Could you check a few things on this model? Use its own coordinates, in mm. Face numbers are marked on the shaded views. A direction names the side the tool comes from. Round coordinates to 2 decimals unless told otherwise and drop trailing zeros. Loops run counter-clockwise (first coordinate to the right, second up) from the corner with the lowest first, then second, coordinate; pieces in that order, holes last. Notation, with made-up numbers: M 30,-32.5 L 66,-32.5 A24 cw 66,4.5 Z; hole C -9,31 d10. An arc over 180 degrees is marked long. One line per item, written item: value. Start each with the question number.
Q1. Imagine slicing it at C-C (x = 80). Please give me the cut outline in (y, z) (3 decimals).
Q2. Which directions (+Z, -Z, +X, -X, +Y, -Y) give clear straight access to the entire face, cutting with the end or side of a thin tool? Please do the marked faces 1, 2 and 3.
Q3. Imagine slicing it at D-D (x = 158). Please give me the cut outline in (y, z).
Q4. Imagine slicing it at A-A (y = 0). Please give me the cut outline in (x, z) (3 decimals), then the cut area to 3 significant figures.
Q5. I'm going to push flat-ended pins straight in: pin 1 Ø12 at (y, z) = (5, 10.5) entering from -X; pin 2 Ø10 at (x, z) = (220, -5.5) entering from +Y; pin 3 Ø1 at (x, y) = (141.5, -11) entering from -Z; pin 4 Ø1.5 at (y, z) = (6, -13) entering from +X. Where does each tip first touch, or does it pass through?
Q6. Please list where these lines run through material, in increasing order: line 1 along Y through (x, z) = (157, -10); line 2 along X through (y, z) = (11.5, -3).
from build123d import *


with BuildPart() as part:
    # Sketch1 → Revolve1 (revolve)
    with BuildSketch(Plane.XY):
        with BuildLine():
            Line((0, 0), (0, 7.5))
            Line((0, 7.5), (18.5, 7.5))
            ThreePointArc((18.5, 7.5), (19.560660172, 7.939339828), (20, 9))
            Line((20, 9), (20, 16.675))
            Line((20, 16.675), (142, 16.675))
            Line((142, 16.675), (142, 14))
            ThreePointArc((142, 14), (142.439339828, 12.939339828), (143.5, 12.5))
            Line((143.5, 12.5), (310, 12.5))
            Line((310, 12.5), (310, 9))
            ThreePointArc((310, 9), (310.439339828, 7.939339828), (311.5, 7.5))
            Line((311.5, 7.5), (330, 7.5))
            Line((330, 7.5), (330, 0))
            Line((330, 0), (0, 0))
        make_face()
    revolve(axis=Axis((330, 0, 0), (-1, 0, 0)))


solid = part.part
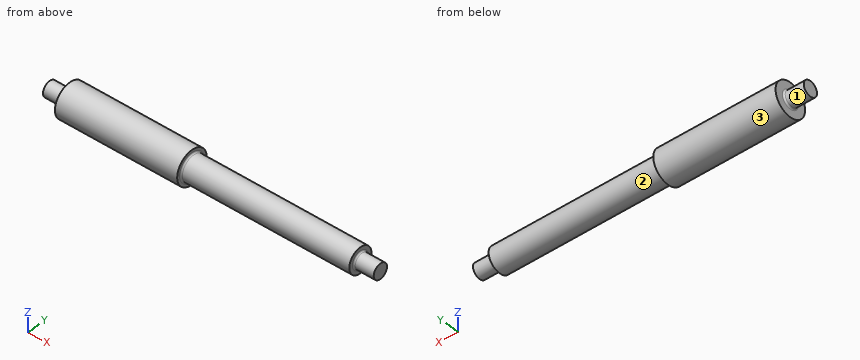
Report:
1. outline: C 0,0 d33.35
2. face 1: -X
2. face 2: +X
2. face 3: +X, -X
3. outline: C 0,0 d25
4. outline: M 0,-7.5 L 18.5,-7.5 A1.5 cw 20,-9 L 20,-16.675 L 142,-16.675 L 142,-14 A1.5 cw 143.5,-12.5 L 310,-12.5 L 310,-9 A1.5 cw 311.5,-7.5 L 330,-7.5 L 330,7.5 L 311.5,7.5 A1.5 cw 310,9 L 310,12.5 L 143.5,12.5 A1.5 cw 142,14 L 142,16.675 L 20,16.675 L 20,9 A1.5 cw 18.5,7.5 L 0,7.5 Z
4. area: 8,870 mm²
5. pin 1: stops at x = 0
5. pin 2: stops at y = 12.49
5. pin 3: stops at z = -12.95
5. pin 4: stops at x = 142.06
6. line 1: y = -7.5 to 7.5
6. line 2: x = 20 to 310
